Verification items for the finished model (mm, model axes). A direction names the side the tool comes from. Coordinates: 2 decimals unless noted, no trailing zeros. Loops run counter-clockwise (first coordinate to the right, second up) from the corner with the lowest first, then second, coordinate; pieces in that order, holes last. Notation, with made-up numbers: M -4.5,20 L 22.5,20 A25 cw 22.5,36 Z; hole C 10,49 d8. An arc over 180 degrees is marked long. Write item = value, one per line. Start each with the question number.
```python
from build123d import *

# Parameters (mm, degrees)
F1_DEPTH = 63.5
F3_DEPTH = 0.5334
F5_DEPTH = 0.5334
F7_DEPTH = 63.5
F8_W     = 22.86
F8_H     = 50.8
F9_DEPTH = 10.16


with BuildPart() as f1:
    # F0 (on Front) → F1 (new body)
    with BuildSketch(Plane.XZ):
        Polygon((0, 30.48), (0, 0), (35.56, 0), (35.56, 8.27462), (35.0266, 8.27462), (35.0266, 0.5334), (0.5334, 0.5334), (0.5334, 30.234671), (17.78, 45.017471), (35.0266, 30.234671), (35.0266, 20.142561), (35.56, 20.142561), (35.56, 30.48), (17.78, 45.72), align=None)
    extrude(amount=F1_DEPTH)

    # F2 (on face) → F3 (join)
    with BuildSketch(Plane.XZ.offset(63.5)):
        Polygon((35.0266, 0.5334), (35.0266, 30.234671), (17.78, 45.017471), (0.5334, 30.234671), (0.5334, 0.5334), align=None)
    extrude(amount=-F3_DEPTH)

    # F4 (on face) → F5 (join)
    with BuildSketch(Plane(origin=(0, 0, 0), x_dir=(-1, 0, 0), z_dir=(0, 1, 0))):
        Polygon((-35.0266, 30.234671), (-35.0266, 0.5334), (-0.5334, 0.5334), (-0.5334, 30.234671), (-17.78, 45.017471), align=None)
    extrude(amount=-F5_DEPTH)

    # F6 (on face) → F7 (join)
    with BuildSketch(Plane.XZ.offset(63.5)):
        Polygon((12.1666, 40.908514), (12.1666, 0), (12.7, 0), (12.7, 41.365714), align=None)
    extrude(amount=-F7_DEPTH)

    # F8 (on Top) → F9 (join)
    with BuildSketch(Plane.XY):
        with Locations((23.5966, -37.5666)):
            Rectangle(F8_W, F8_H)
    extrude(amount=F9_DEPTH)


solid = f1.part
```
Q1. Gauge pin test, flat ends, axial feed: pin 1 (6 mm diameter, centred on x = 9.5, z = 29, fed in from +Y); pin 2 (9.5 mm diameter, centred on x = 25, y = -5, fed in from +Z); pin 3 (6 mm diameter, centred on y = -24, z = 12, fed in from +X); pin 4 (3.5 mm diameter, centred on x = 7, y = -16.5, fed in from +Z). Record the tip position at first contact, or that the pin passes through.
Q2. Set-up check for faces 1 (the face through (24, -37, 10.16)), 2 (the face through (35.56, -31, 25)), 3 (the face through (35.027, -38, 9)), 4 (the face through (6, -62.967, 16)): record each of +Z, -Z, +X, -X, +Y, -Y from which the full face is reachable in a straight line by a thin tool's end or side.
Q3. Sectioned sample at A-A on y = -21.5. Record the cut outline in (x, z), plus the area to 3 significant figures.
Q4. Sectioned sample at B-B on x = 23.5. Record the cut outline in (y, z), plus the area to 3 significant figures.
Q5. Mould release check, pull along Y, two halves, no side actions. Record for faces 5 (the face through (0, -31, 15)), 6 (the face through (18, 0, 18)), 7 (the face through (24, -0.533, 18)): +Y half, -Y half, draft (parallel to the pull), parting line (faces both ways), or undercut.
Q6. Sectioned sample at C-C on z = 37. Record the cut outline in (x, y).
Q7. Sectioned sample at D-D on z = 43.5. Record the cut outline in (x, y).
Q8. Scan lines: L1, parallel to X at y = -26.5, z = 26.5; L2, parallel to Y at x = 7.5, z = 35.5; L3, parallel to X at y = -35, z = 34. Record each from-to range of solid material in increasing order. Write a range as [from, to].
Solutions:
q1.pin_1 = 0
q1.pin_2 = 43.6
q1.pin_3 = 35.03
q1.pin_4 = 37.98
q2.face_1 = +X
q2.face_2 = +Z, -Z, +X, +Y, -Y
q2.face_3 = +X, +Y, -Y
q2.face_4 = none
q3.outline = M 0,0 L 35.56,0 L 35.56,8.27 L 35.03,8.27 L 35.03,10.16 L 12.7,10.16 L 12.7,40.66 L 17.78,45.02 L 35.03,30.23 L 35.03,20.14 L 35.56,20.14 L 35.56,30.48 L 17.78,45.72 L 0,30.48 Z; hole M 0.53,0.53 L 12.17,0.53 L 12.17,40.21 L 0.53,30.23 Z
q3.area = 305 mm²
q4.outline = M -63.5,0 L 0,0 L 0,40.82 L -63.5,40.82 Z; hole M -62.97,10.16 L -12.17,10.16 L -12.17,0.53 L -0.53,0.53 L -0.53,40.11 L -62.97,40.11 Z
q4.area = 610 mm²
q5.face_5 = draft
q5.face_6 = +Y half
q5.face_7 = undercut
q6.outline = M 7.61,-63.5 L 27.95,-63.5 L 27.95,0 L 7.61,0 Z; hole M 8.43,-62.97 L 12.17,-62.97 L 12.17,-0.53 L 8.43,-0.53 Z; hole M 12.7,-62.97 L 27.13,-62.97 L 27.13,-0.53 L 12.7,-0.53 Z
q7.outline = M 15.19,-63.5 L 20.37,-63.5 L 20.37,0 L 15.19,0 Z; hole M 16.01,-62.97 L 19.55,-62.97 L 19.55,-0.53 L 16.01,-0.53 Z
q8.L1 = [0, 0.53], [12.17, 12.7], [35.03, 35.56]
q8.L2 = [-63.5, -62.97], [-0.53, 0]
q8.L3 = [4.11, 4.93], [12.17, 12.7], [30.63, 31.45]
